Check sheet for the modelled part. Datum: model origin and axes. Units: mm. Give positions to 0.01 mm unless a question says otherwise; leave off trailing zeros. Order: outer loops, then holes, each group sorted by start corner. A loop starts at its lowest first (then second) coordinate and runs counter-clockwise, first axis right, second up. Notation, with made-up numbers: (55.25, 11) -> (60.25, 11) arc R30 cw to (60.25, 42) -> close; hole circle Ø10 at (42, 75.5). An arc over 180 degrees is marked (long way). Answer in a Markdown table with one row per item. Add a question column.
(1) Cross-section at C-C (z = 54). Record the cut outline in (x, y), then the cut area to 3 significant figures.
(2) Cross-section at B-B (y = 0). Record the cut outline in (x, z).
(3) Thickness scan on L1, parallel to X at y = 0, z = 76; L2, parallel to X at y = 6.25, z = 166; L3, parallel to Y at x = -5.25, z = 46. Record the ranges inside material, lowest first. Write a range as [from, to].
(4) Cross-section at A-A (x = 0). Record the cut outline in (y, z).
(5) Cross-section at D-D (z = 79.5). Record the cut outline in (x, y).
(6) Go/stop test with flat-tipped pins: pin 1 (1.5 mm diameter, centred on x = -1.5, z = 107, fed in from -Y); pin 2 (1.5 mm diameter, centred on y = -6.5, z = 35, fed in from -X); pin 3 (3.5 mm diameter, centred on x = 0, z = 54, fed in from +Y); pin 4 (1.5 mm diameter, centred on x = 1.5, z = 25.5, fed in from +Y). Record where each tip stops, or that it passes through.
```python
from build123d import *

# Parameters (mm, degrees)
F0_R     = 8
F0_R_2   = 7
F1_DEPTH = 190
F2_R     = 3
F3_DEPTH = 20
F4_R     = 3
F5_DEPTH = 12.5


with BuildPart() as f1:
    # F0 (on Top) → F1 (new body)
    with BuildSketch(Plane.XY):
        Circle(F0_R)
        Circle(F0_R_2, mode=Mode.SUBTRACT)
    extrude(amount=F1_DEPTH)

    # F2 (on Right) → F3 (cut, symmetric)
    with BuildSketch(Plane.YZ):
        with Locations((0, 44)):
            Circle(F2_R)
    extrude(amount=F3_DEPTH, both=True, mode=Mode.SUBTRACT)

    # F4 (on Front) → F5 (cut, symmetric)
    with BuildSketch(Plane.XZ):
        with Locations((0, 54)):
            Circle(F4_R)
    extrude(amount=F5_DEPTH, both=True, mode=Mode.SUBTRACT)


solid = f1.part
```
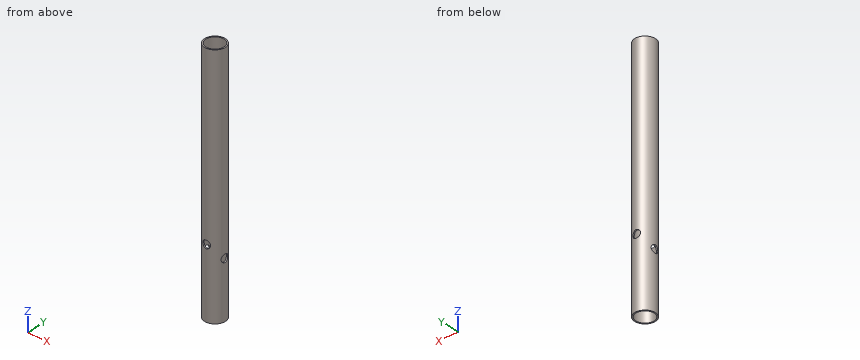
Answer below:
| question | item | result |
|---|---|---|
| 1 | outline | (-3, -7.42) -> (-3, -6.32) arc R7 cw to (-3, 6.32) -> (-3, 7.42) arc R8 ccw to start; (3, -7.42) arc R8 ccw to (3, 7.42) -> (3, 6.32) arc R7 cw to (3, -6.32) -> close |
| 1 | area | 34.8 mm² |
| 2 | outline | (-8, 0) -> (-7, 0) -> (-7, 41) -> (-8, 41) -> close; (-8, 47) -> (-7, 47) -> (-7, 190) -> (-8, 190) -> close; (7, 0) -> (8, 0) -> (8, 41) -> (7, 41) -> close; (7, 47) -> (8, 47) -> (8, 190) -> (7, 190) -> close |
| 3 | L1 | x = [-8, -7], [7, 8] |
| 3 | L2 | x = [-4.99, -3.15], [3.15, 4.99] |
| 3 | L3 | y = [-6.04, -4.63], [4.63, 6.04] |
| 4 | outline | (-8, 0) -> (-7, 0) -> (-7, 51) -> (-8, 51) -> close; (-8, 57) -> (-7, 57) -> (-7, 190) -> (-8, 190) -> close; (7, 0) -> (8, 0) -> (8, 51) -> (7, 51) -> close; (7, 57) -> (8, 57) -> (8, 190) -> (7, 190) -> close |
| 5 | outline | circle Ø16 at (0, 0); hole circle Ø14 at (0, 0) |
| 6 | pin 1 | stops at y = -7.96 |
| 6 | pin 2 | stops at x = -5.56 |
| 6 | pin 3 | passes through |
| 6 | pin 4 | stops at y = 7.96 |
